Geometry check sheet. Reference: the model listing, model coordinates, mm. Round coordinates to 2 decimals unless told otherwise and drop trailing zeros. Order: outer loops, then holes, each group sorted by start corner. A loop starts at its lowest first (then second) coordinate and runs counter-clockwise, first axis right, second up. Notation, with made-up numbers: (-30, -27) - (-22, -27) arc R28 cw to (-22, -3) - close; hole circle Ø10 at (51, 22.25). An arc over 180 degrees is marked (long way). Return JSON: item names as keys, results as strings. Group by question number.
Q1. Sectioned sample at A-A, the plane y = 0. Record the cut outline in (x, z), then the cut area to 3 significant figures.
Q2. Material ranges on line 1 along Z through (x, y) = (-58, 0); line 2 along Y through (x, z) = (-1, 6); line 3 along X through (y, z) = (7.5, -5.25), recorded low to high.
Q3. Gauge pin test, flat ends, axial feed: pin 1 Ø1.5 at (y, z) = (47, -4) entering from -X; pin 2 Ø5 at (y, z) = (0, 0) entering from -X; pin 3 Ø3.5 at (x, z) = (0, 0) entering from -Y; pin 4 Ø2.5 at (x, z) = (0, 0) entering from +Y. Record the tip position at first contact, or that the pin passes through.
Q4. Sectioned sample at C-C, the plane z = -3.5. Record the cut outline in (x, y), then the cut area to 3 significant figures.
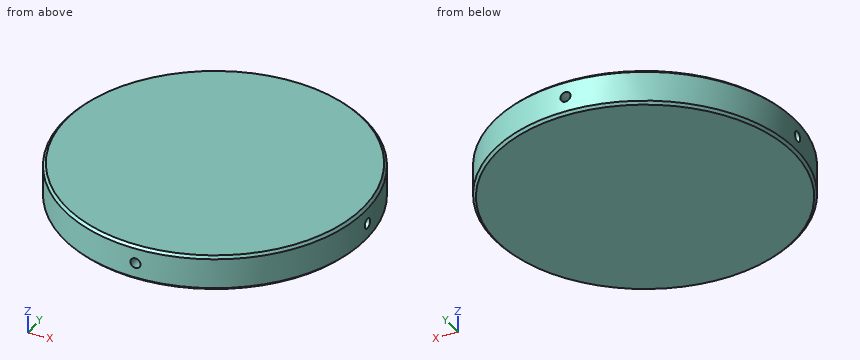
```python
from build123d import *

# Parameters (mm, degrees)
SKETCH1_R           = 60
BOSS_EXTRUDE1_DEPTH = 7
CHAMFER1_SIZE       = 1
CUT_EXTRUDE1_START  = 55
SKETCH2_R           = 2
CUT_EXTRUDE1_DEPTH  = 10
CUT_EXTRUDE2_START  = -65
SKETCH2_2_R         = 2
CUT_EXTRUDE2_DEPTH  = 10
CUT_EXTRUDE3_START  = 55
SKETCH3_R           = 2
CUT_EXTRUDE3_DEPTH  = 10
CUT_EXTRUDE4_START  = -65
SKETCH3_2_R         = 2
CUT_EXTRUDE4_DEPTH  = 10


with BuildPart() as part:
    # Sketch1 → Boss-Extrude1 (new, symmetric)
    with BuildSketch(Plane.XY):
        Circle(SKETCH1_R)
    extrude(amount=BOSS_EXTRUDE1_DEPTH, both=True)

    # Chamfer1
    chamfer1_edges = [part.edges().sort_by_distance(p)[0] for p in [
        (-60, 0, -7),
        (-60, 0, 7),
    ]]
    chamfer(chamfer1_edges, length=CHAMFER1_SIZE)

    # Sketch2 → Cut-Extrude1 (cut)
    with BuildSketch(Plane(origin=(0, 0, 0), x_dir=(1, 0, 0), z_dir=(0, 1, 0)).offset(CUT_EXTRUDE1_START)):
        with Locations(Location((0, 0, 0), (0, 0, 90))):
            Circle(SKETCH2_R)
    extrude(amount=CUT_EXTRUDE1_DEPTH, mode=Mode.SUBTRACT)

    # Sketch2_2 → Cut-Extrude2 (cut)
    with BuildSketch(Plane(origin=(0, 0, 0), x_dir=(1, 0, 0), z_dir=(0, 1, 0)).offset(CUT_EXTRUDE2_START)):
        with Locations(Location((0, 0, 0), (0, 0, 90))):
            Circle(SKETCH2_2_R)
    extrude(amount=CUT_EXTRUDE2_DEPTH, mode=Mode.SUBTRACT)

    # Sketch3 → Cut-Extrude3 (cut)
    with BuildSketch(Plane(origin=(0, 0, 0), x_dir=(0, 0, -1), z_dir=(1, 0, 0)).offset(CUT_EXTRUDE3_START)):
        Circle(SKETCH3_R)
    extrude(amount=CUT_EXTRUDE3_DEPTH, mode=Mode.SUBTRACT)

    # Sketch3_2 → Cut-Extrude4 (cut)
    with BuildSketch(Plane(origin=(0, 0, 0), x_dir=(0, 0, -1), z_dir=(1, 0, 0)).offset(CUT_EXTRUDE4_START)):
        Circle(SKETCH3_2_R)
    extrude(amount=CUT_EXTRUDE4_DEPTH, mode=Mode.SUBTRACT)


solid = part.part
```
Reply:
{
 "1": {"outline": "(-60, -6) - (-59, -7) - (59, -7) - (60, -6) - (60, -2) - (55, -2) - (55, 2) - (60, 2) - (60, 6) - (59, 7) - (-59, 7) - (-60, 6) - (-60, 2) - (-55, 2) - (-55, -2) - (-60, -2) - close", "area": "1,640 mm^2"},
 "2": {"line 1": "-7 to -2, 2 to 7", "line 2": "-59.99 to 59.99", "line 3": "-59.53 to 59.53"},
 "3": {"pin 1": "x = -38.22", "pin 2": "x = -60", "pin 3": "y = -55", "pin 4": "y = 55"},
 "4": {"outline": "circle Ø120 at (0, 0)", "area": "11,300 mm^2"}
}
